from build123d import *

# Parameters (mm, degrees)
SKETCH1_W           = 50
SKETCH1_H           = 25
BOSS_EXTRUDE1_DEPTH = 49
CUT_EXTRUDE2_DEPTH  = 55
SKETCH5_R           = 1.25
SKETCH5_W           = 19.5
SKETCH5_H           = 12
CUT_EXTRUDE3_DEPTH  = 12.5
SKETCH7_W           = 50
SKETCH7_H           = 49
CUT_EXTRUDE4_DEPTH  = 8
CHAMFER1_SIZE       = 1
SKETCH8_W           = 17.539951448
SKETCH8_H           = 49.569428005
CUT_EXTRUDE5_DEPTH  = 12.5
CHAMFER2_SIZE       = 1
SKETCH9_R           = 3.75
CUT_EXTRUDE6_DEPTH  = 4


with BuildPart() as part:
    # Sketch1 → Boss-Extrude1 (new body)
    with BuildSketch(Plane(origin=(0, 0, 0), x_dir=(1, 0, 0), z_dir=(0, 1, 0))):
        with Locations((25, 12.5)):
            Rectangle(SKETCH1_W, SKETCH1_H)
    extrude(amount=BOSS_EXTRUDE1_DEPTH)

    # Sketch4 → Cut-Extrude2 (cut)
    with BuildSketch(Plane(origin=(50, 0, 0), x_dir=(0, 0, -1), z_dir=(1, 0, 0))):
        Polygon((9.775, 45), (16.125, 45), (16.125, 34.127502784), (16.125, 12.627502784), (16.125, 4), (9.775, 4), (9.775, 13.75), (9.775, 35.25), align=None)
    extrude(amount=-CUT_EXTRUDE2_DEPTH, mode=Mode.SUBTRACT)

    # Sketch5 → Cut-Extrude3 (cut)
    with BuildSketch(Plane(origin=(0, 0, -25), x_dir=(-1, 0, 0), z_dir=(0, 0, -1))):
        with Locations((-32.5, 24.5)):
            Circle(SKETCH5_R)
        with Locations((-7.5, 24.5)):
            Circle(SKETCH5_R)
        with Locations((-20, 24.5)):
            Rectangle(SKETCH5_W, SKETCH5_H)
    extrude(amount=-CUT_EXTRUDE3_DEPTH, mode=Mode.SUBTRACT)

    # Sketch7 → Cut-Extrude4 (cut)
    with BuildSketch(Plane.XY):
        with Locations((25, 24.5)):
            Rectangle(SKETCH7_W, SKETCH7_H)
    extrude(amount=-CUT_EXTRUDE4_DEPTH, mode=Mode.SUBTRACT)

    # Chamfer1
    chamfer1_edges = [part.edges().sort_by_distance(p)[0] for p in [
        (25, 49, -25),
        (0, 49, -16.5),
        (25, 0, -25),
        (0, 0, -16.5),
        (50, 0, -16.5),
        (50, 49, -16.5),
        (0, 24.5, -8),
        (25, 49, -8),
        (50, 24.5, -8),
        (25, 0, -8),
        (0, 24.5, -25),
        (50, 24.5, -25),
    ]]
    chamfer(chamfer1_edges, length=CHAMFER1_SIZE)

    # Sketch8 → Cut-Extrude5 (cut)
    with BuildSketch(Plane(origin=(50, 0, 0), x_dir=(0, 0, -1), z_dir=(1, 0, 0))):
        with Locations((16.404674177, 24.368191016)):
            Rectangle(SKETCH8_W, SKETCH8_H)
    extrude(amount=-CUT_EXTRUDE5_DEPTH, mode=Mode.SUBTRACT)

    # Chamfer2
    # the kernel refuses this chamfer: 1 mm, written as the material it takes off along each edge
    with BuildSketch(Plane(origin=(37.5, 0, -6.428317012), x_dir=(-0.9996219169112968, -0.027495876610586292, 0), z_dir=(0, 0, -1))) as chamfer2_piece_1:
        Polygon((CHAMFER2_SIZE * 0.999621916911, CHAMFER2_SIZE * 0.0274958766106), (-CHAMFER2_SIZE * 0.0274958766106, CHAMFER2_SIZE * 0.999621916911), (0, 0), align=None)
    extrude(amount=20.143365976, mode=Mode.SUBTRACT)
    with BuildSketch(Plane(origin=(37.5, 49, -6.428317012), x_dir=(-0.9996219169112968, 0.027495876610589005, 0), z_dir=(0, 0, -1))) as chamfer2_piece_2:
        Polygon((CHAMFER2_SIZE * 0.999621916911, -CHAMFER2_SIZE * 0.0274958766106), (-CHAMFER2_SIZE * 0.0274958766106, -CHAMFER2_SIZE * 0.999621916911), (0, 0), align=None)
    extrude(amount=20.143365976, mode=Mode.SUBTRACT)
    with BuildSketch(Plane(origin=(37.5, 50.571682988, -8), x_dir=(-0.9996219169112968, 0, 0.027495876610586414), z_dir=(0, -1, 0)), Plane(origin=(37.5, -1.571682988, -25), x_dir=(-0.9996219169112968, 0, -0.02749587661058555), z_dir=(0, 1, 0))) as chamfer2_piece_3:
        Polygon((CHAMFER2_SIZE * 0.999621916911, CHAMFER2_SIZE * 0.0274958766106), (-CHAMFER2_SIZE * 0.0274958766106, CHAMFER2_SIZE * 0.999621916911), (0, 0), align=None)
    extrude(amount=52.143365976, mode=Mode.SUBTRACT)

    # Sketch9 → Cut-Extrude6 (cut)
    with BuildSketch(Plane.XY.offset(-8)):
        with Locations((18.75, 24.5)):
            Circle(SKETCH9_R)
    extrude(amount=-CUT_EXTRUDE6_DEPTH, mode=Mode.SUBTRACT)


solid = part.part
Design review of the part built by this model. Coordinates are the model's own, in mm. A direction names the side the tool comes from. Coordinates: 2 decimals unless noted, no trailing zeros. Write each loop counter-clockwise with the first axis right and the second up, starting at its lowest first coordinate (ties: lowest second). Pieces come first, ordered by that corner, then holes. Notation, with made-up numbers: (6.5, 41.25) -> (20.5, 41.25) arc R9 ccw to (20.5, 51.25) -> close; hole circle Ø5 at (63, -18.5). An arc over 180 degrees is marked (long way). Write each question's results on one line, items separated by ' | '. Start each with the question number.
(1) For line 1 along Z through (x, y) = (30, 40) (3 decimals); line 2 along Y through (x, z) = (16.5, -18.75); line 3 along Y through (x, z) = (32.5, -14.75), list the stretches that pass through material, from the lowest coordinate up. Write a range as from..to.
(2) Clearance check with a flat-ended pin moving along its axis: P1, Ø10, axis at x = 18.75, y = 24.5, coming from the -Z side (3 decimals). State where the tip first meets the part, or that it passes through.
(3) Take a section at D-D on z = -13.75. Write out the cut boundary in (x, y), and give its area (3 significant figures).
(4) Take a section at B-B on y = 24.5. Write out the cut boundary in (x, z) (3 decimals), and give its area (3 significant figures).
(5) Take a section at C-C on x = 34.5. Write out the cut boundary in (y, z) (3 decimals).
(6) Take a section at A-A on x = 18.75. Write out the cut boundary in (y, z) (3 decimals), and give its area (3 significant figures).
(7) The part is to be moulded in two halves that separate along Z. For faces 1 (the face through (19, 45, -13)), 2 (the face through (18.7, 0.5, -8.5)), 3 (the face through (10.25, 24, -21)), say which applies: pulls with the +Z half, pulls with the -Z half, needs draft (parallel to the pull), parting line crosses it, or undercut.
(8) Tool access review of faces 4 (the face through (19, 4, -13)), 5 (the face through (0.7, 0.7, -8.6)), 6 (the face through (29.75, 24, -21)): name each direction out of +Z, -Z, +X, -X, +Y, -Y from which nothing blocks a thin tool from reaching the whole face with its end or side.
Results found:
1) line 1: z = -25..-16.125, -9.775..-8 | line 2: y = 0..18.5, 30.5..49 | line 3: y = 0..4, 45..49
2) P1: stops at z = -9.775
3) outline: (0, 1) -> (1, 0) -> (36.5, 0) -> (37.5, 1) -> (37.5, 4) -> (0, 4) -> close; (0, 45) -> (37.5, 45) -> (37.5, 48) -> (36.5, 49) -> (1, 49) -> (0, 48) -> close | area: 298 mm2
4) outline: (0, -24) -> (1, -25) -> (6.25, -25) -> (6.25, -16.125) -> (0, -16.125) -> close; (0, -9.775) -> (15, -9.775) -> (15, -8) -> (1, -8) -> (0, -9) -> close; (8.75, -25) -> (10.25, -25) -> (10.25, -16.125) -> (8.75, -16.125) -> close; (22.5, -9.775) -> (37.5, -9.775) -> (37.5, -9) -> (36.5, -8) -> (22.5, -8) -> close; (29.75, -25) -> (31.25, -25) -> (31.25, -16.125) -> (29.75, -16.125) -> close; (33.75, -25) -> (36.5, -25) -> (37.5, -24) -> (37.5, -16.125) -> (33.75, -16.125) -> close | area: 167 mm2
5) outline: (0, -24) -> (1, -25) -> (48, -25) -> (49, -24) -> (49, -9) -> (48, -8) -> (1, -8) -> (0, -9) -> close; hole (4, -16.125) -> (45, -16.125) -> (45, -9.775) -> (4, -9.775) -> close
6) outline: (0, -24) -> (1, -25) -> (18.5, -25) -> (18.5, -16.125) -> (4, -16.125) -> (4, -9.775) -> (20.75, -9.775) -> (20.75, -8) -> (1, -8) -> (0, -9) -> close; (28.25, -9.775) -> (45, -9.775) -> (45, -16.125) -> (30.5, -16.125) -> (30.5, -25) -> (48, -25) -> (49, -24) -> (49, -9) -> (48, -8) -> (28.25, -8) -> close | area: 451 mm2
7) face 1: undercut | face 2: pulls with the +Z half | face 3: needs draft
8) face 4: +X, -X | face 5: +Z, -X, -Y | face 6: -Z
